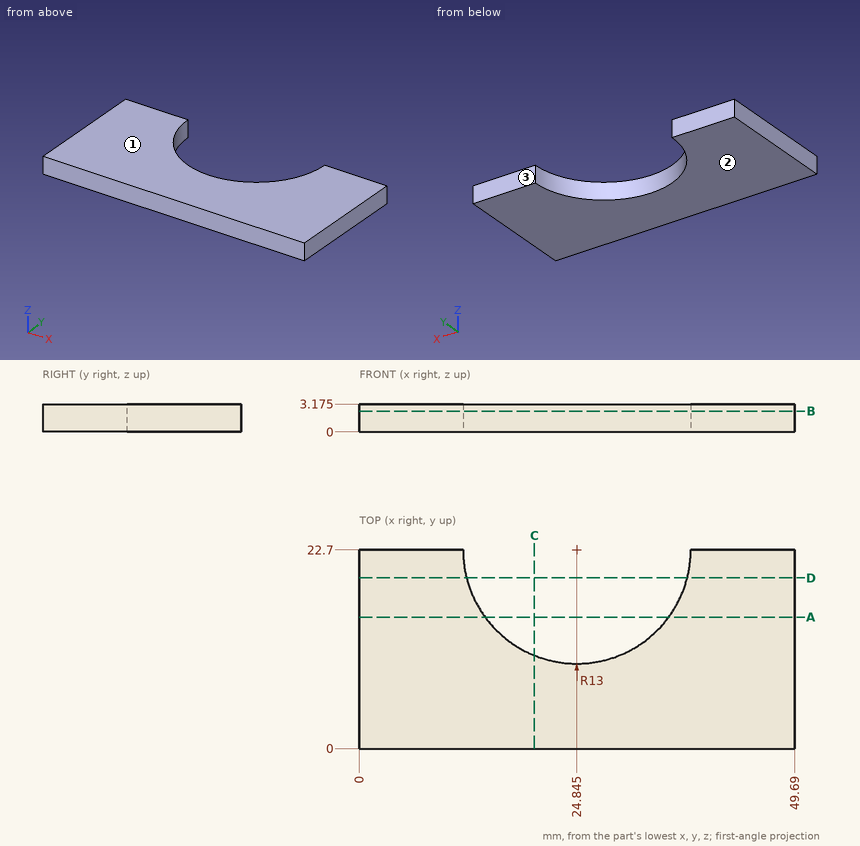
Answer from the drawing. Dimensions are ordinates in mm from the lowest x, y and z of the part. Give positions to 0.01 mm unless a question says otherwise; leave off trailing zeros. Loops run counter-clockwise (first coordinate to the right, second up) from the corner with the lowest first, then second, coordinate; pieces in that order, holes last. Notation, with made-up numbers: (88.5, 69.25) - (105.5, 69.25) arc R21 ccw to (105.5, 78.25) - close; hole circle Ø4 at (80, 81). An arc over 180 degrees is marked (long way). Answer as a JSON object with one key per item and string values.
1. For a pull along Z with two mould halves and no side action, classify the marked faces 1, 2 and 3 as pulls with the +Z half, pulls with the -Z half, needs draft (parallel to the pull), parting line crosses it, or undercut.
Determined:
{"face 1": "pulls with the +Z half", "face 2": "pulls with the -Z half", "face 3": "needs draft"}
2. A cutting plane is placed at B-B (z = 2.35). Write down the section's boundary in (x, y) (3 decimals), then the cut area to 4 significant figures.
Determined:
{"outline": "(0, 0) - (49.69, 0) - (49.69, 22.7) - (37.845, 22.7) arc R13 cw to (11.845, 22.7) - (0, 22.7) - close", "area": "862.5 mm²"}
3. A cutting plane is placed at C-C (x = 20). Write down the section's boundary in (y, z) (3 decimals), then the cut area to 3 significant figures.
Determined:
{"outline": "(0, 0) - (10.637, 0) - (10.637, 3.175) - (0, 3.175) - close", "area": "33.8 mm²"}
4. Find the intervals of material crossed by L1, parallel to X at y = 17.75, z = 2.6; L2, parallel to X at y = 20, z = 0.5; L3, parallel to Y at x = 15, z = 0.55, in increasing order. Write a range as [from, to].
Determined:
{"L1": "[0, 12.82], [36.87, 49.69]", "L2": "[0, 12.13], [37.56, 49.69]", "L3": "[0, 14.21]"}
5. A cutting plane is placed at A-A (y = 15). Write down the section's boundary in (x, z) (3 decimals).
Determined:
{"outline": "(0, 0) - (14.371, 0) - (14.371, 3.175) - (0, 3.175) - close; (35.319, 0) - (49.69, 0) - (49.69, 3.175) - (35.319, 3.175) - close"}
6. A cutting plane is placed at D-D (y = 19.5). Write down the section's boundary in (x, z) (3 decimals).
Determined:
{"outline": "(0, 0) - (12.245, 0) - (12.245, 3.175) - (0, 3.175) - close; (37.445, 0) - (49.69, 0) - (49.69, 3.175) - (37.445, 3.175) - close"}
